For this review, take the finished solid that the model builds, in its own axes (mm). Give positions to 0.01 mm unless a question says otherwise; leave off trailing zeros. Loops run counter-clockwise (first coordinate to the right, second up) from the corner with the lowest first, then second, coordinate; pieces in that order, holes last. Notation, with made-up numbers: (74, -31.5) -> (78, -31.5) arc R25 cw to (78, -17.5) -> close; hole circle Ø6 at (37, 62). An arc over 180 degrees is marked (long way). Write each question's results on one line, items separated by ' | '. Start each with the question number.
```python
from build123d import *

# Parameters (mm, degrees)
SKETCH_1_W          = 61
SKETCH_1_H          = 42
SKETCH_1_R          = 1.75
EXTRUDE_1_DEPTH     = 2
EXTRUDE_2_DEPTH     = 2
SKETCH_3_OUTSIDE_W  = 82.34
SKETCH_3_OUTSIDE_H  = 96.34
CUT_EXTRUDE_1_DEPTH = 10


with BuildPart() as part:
    # 草图1 → 凸台-拉伸1 (new body)
    with BuildSketch(Plane.XY):
        with Locations((30.5, 21)):
            Rectangle(SKETCH_1_W, SKETCH_1_H)
        with Locations((20, 3)):
            Circle(SKETCH_1_R, mode=Mode.SUBTRACT)
        with Locations((40, 3)):
            Circle(SKETCH_1_R, mode=Mode.SUBTRACT)
        with Locations(Location((40, 39, 0), (0, 0, 180))):
            Circle(SKETCH_1_R, mode=Mode.SUBTRACT)
        with Locations(Location((20, 39, 0), (0, 0, 180))):
            Circle(SKETCH_1_R, mode=Mode.SUBTRACT)
    extrude(amount=EXTRUDE_1_DEPTH)

    # 草图2 → 凸台-拉伸2 (add)
    with BuildSketch(Plane.XY.offset(2)):
        Polygon((61, 75), (0, 42), (61, 42), align=None)
    extrude(amount=-EXTRUDE_2_DEPTH)

    # 草图3 outside → 切除-拉伸1 (cut)
    with BuildSketch(Plane.XY.offset(2)):
        with Locations((30.5, 37.5)):
            Rectangle(SKETCH_3_OUTSIDE_W, SKETCH_3_OUTSIDE_H)
        with BuildLine():
            Line((0, 41.106045159), (0, 1.5))
            ThreePointArc((0, 1.5), (0.439339828, 0.439339828), (1.5, 0))
            Line((1.5, 0), (59.5, 0))
            ThreePointArc((59.5, 0), (60.560660172, 0.439339828), (61, 1.5))
            Line((61, 1.5), (61, 72.483094339))
            ThreePointArc((61, 72.483094339), (60.26792193, 73.771619042), (58.786272122, 73.802409508))
            Line((58.786272122, 73.802409508), (0.786272122, 42.425360328))
            ThreePointArc((0.786272122, 42.425360328), (0.211475298, 41.873967089), (0, 41.106045159))
        make_face(mode=Mode.SUBTRACT)
    extrude(amount=-CUT_EXTRUDE_1_DEPTH, mode=Mode.SUBTRACT)


solid = part.part
```
1. Draft analysis for pull direction X (two halves, no side actions). For faces 1 (the flat face through (61, 36, 1)), 2 (the cylindrical face through (60.29, 73.76, 1.01)), 3 (the cylindrical face through (38.383, 39.67, 0.986)), 4 (the cylindrical face through (0.43, 0.45, 1.01)), state which applies: released by +X, released by -X, zero draft, split by the parting line, or undercut.
2. We need section D-D (y = 58). Write out the cut boundary in (x, z).
3. We need section C-C (x = 40). Write out the cut boundary in (y, z).
4. We need section B-B (z = 1.55). Write out the cut boundary in (x, y), plus the area to 3 significant figures.
5. We need section A-A (y = 39). Write out the cut boundary in (x, z).
6. Wall thickness on L1, parallel to Y at x = 20, z = 0.95; L2, parallel to Y at x = 40, z = 1.5; L3, parallel to X at y = 40, z = 0.3: over which ranges is each line inside the solid? List them lowest first.
Response:
1) face 1: released by +X | face 2: split by the parting line | face 3: undercut | face 4: released by -X
2) outline: (29.58, 0) -> (61, 0) -> (61, 2) -> (29.58, 2) -> close
3) outline: (0, 0) -> (1.25, 0) -> (1.25, 2) -> (0, 2) -> close; (4.75, 0) -> (37.25, 0) -> (37.25, 2) -> (4.75, 2) -> close; (40.75, 0) -> (63.64, 0) -> (63.64, 2) -> (40.75, 2) -> close
4) outline: (0, 1.5) arc R1.5 ccw to (1.5, 0) -> (59.5, 0) arc R1.5 ccw to (61, 1.5) -> (61, 72.48) arc R1.5 ccw to (58.79, 73.8) -> (0.79, 42.43) arc R1.5 ccw to (0, 41.11) -> close; hole circle Ø3.5 at (20, 3); hole circle Ø3.5 at (20, 39); hole circle Ø3.5 at (40, 3); hole circle Ø3.5 at (40, 39) | area: 3,530 mm2
5) outline: (0, 0) -> (18.25, 0) -> (18.25, 2) -> (0, 2) -> close; (21.75, 0) -> (38.25, 0) -> (38.25, 2) -> (21.75, 2) -> close; (41.75, 0) -> (61, 0) -> (61, 2) -> (41.75, 2) -> close
6) L1: y = 0 to 1.25, 4.75 to 37.25, 40.75 to 52.82 | L2: y = 0 to 1.25, 4.75 to 37.25, 40.75 to 63.64 | L3: x = 0 to 18.56, 21.44 to 38.56, 41.44 to 61
